Read the model definition and answer for the solid it produces. Units are mm, in the model's axes. Give positions to 0.01 mm unless a question says otherwise; leave off trailing zeros. Loops run counter-clockwise (first coordinate to the right, second up) from the corner with the lowest first, then second, coordinate; pieces in that order, holes last. Notation, with made-up numbers: (51.25, -5.5) - (57.25, -5.5) arc R16 ccw to (57.25, 14.5) - close; hole circle Ø9 at (35.25, 51.5). An arc over 180 degrees is marked (long way). Write item = value, one per line.
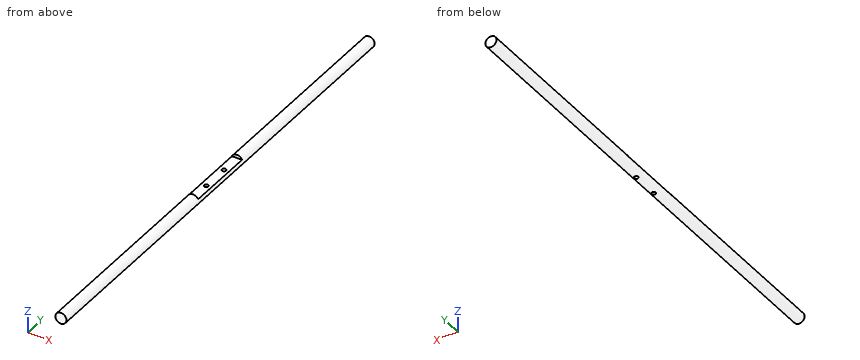
```python
from build123d import *

# Parameters (mm, degrees)
F0_R     = 8
F1_DEPTH = 700
F2_W     = 100
F2_H     = 5
F3_DEPTH = 88
F4_R     = 3
F5_DEPTH = 15


with BuildPart() as f1:
    # F0 (on Front) → F1 (new body)
    with BuildSketch(Plane.XZ):
        with Locations((-65.652847, 44.169296)):
            Circle(F0_R)
    extrude(amount=F1_DEPTH)

    # F2 (on Right) → F3 (cut)
    with BuildSketch(Plane.YZ):
        with Locations((-350, 49.991539)):
            Rectangle(F2_W, F2_H)
    extrude(amount=-F3_DEPTH, mode=Mode.SUBTRACT)

    # F4 (on face) → F5 (cut)
    with BuildSketch(Plane.XY.offset(47.491539)):
        with Locations((-65.344319, -370)):
            Circle(F4_R)
        with Locations((-65.344319, -330)):
            Circle(F4_R)
    extrude(amount=-F5_DEPTH, mode=Mode.SUBTRACT)


solid = f1.part
```
1) A cutting plane is placed at A-A on z = 40.5. Determine the outline of the cut face in (x, y), then the cut area to 3 significant figures.
Output:
outline = (-72.76, -700) - (-58.54, -700) - (-58.54, 0) - (-72.76, 0) - close; hole circle Ø6 at (-65.34, -370); hole circle Ø6 at (-65.34, -330)
area = 9,900 mm²
2) Find the intervals of material crossed by probe 1 along Y at (x, z) = (-60, 49.75); probe 2 along X at (y, z) = (-96, 41); probe 3 along Z at (x, y) = (-65.5, -310), in increasing order.
Output:
probe_1 = -700 to -400, -300 to 0
probe_2 = -73 to -58.31
probe_3 = 36.17 to 47.49
3) Each of these flat-tipped pins is pushed along its axis until it touches: P1, Ø9.5, axis at x = -65.34, y = -330, coming from the +Z side; P2, Ø1.5, axis at y = -240.5, z = 47, coming from the +X side; P3, Ø3, axis at y = -238, z = 46.5, coming from the +X side. Where does it stop, or does it pass through?
Output:
P1 = 47.49
P2 = -57.93
P3 = -57.7
4) A cutting plane is placed at B-B on y = -595. Determine the outline of the cut face in (x, z).
Output:
outline = circle Ø16 at (-65.65, 44.17)
